```python
from build123d import *

# Parameters (mm, degrees)
BOSS_EXTRUDE1_DEPTH = 1.2
SKETCH2_W           = 8.848528138
SKETCH2_H           = 1.5
BOSS_EXTRUDE2_DEPTH = 1.2


with BuildPart() as part:
    # Sketch1 → Boss-Extrude1 (new body)
    with BuildSketch(Plane.XY):
        Polygon((4, 16.152543264), (-4, 16.152543264), (-20.152543264, 0), (0, -20.152543264), (20.152543264, 0), align=None)
        Polygon((-4.424264069, 16.152543264), (-4.624264069, 15.952543264), (-4.482842712, 15.952543264), (-20.435385976, 0), (0, -20.435385976), (20.435385976, 0), (4.482842712, 15.952543264), (4.624264069, 15.952543264), (4.424264069, 16.152543264), (4, 16.152543264), (20.152543264, 0), (0, -20.152543264), (-20.152543264, 0), (-4, 16.152543264), align=None)
        Polygon((-20.435385976, 0), (-4.482842712, 15.952543264), (-4.624264069, 15.952543264), (-20.576807333, 0), (0, -20.576807333), (20.576807333, 0), (4.624264069, 15.952543264), (4.482842712, 15.952543264), (20.435385976, 0), (0, -20.435385976), align=None)
    extrude(amount=BOSS_EXTRUDE1_DEPTH)

    # Sketch2 → Boss-Extrude2 (add)
    with BuildSketch(Plane.XY):
        with Locations((0, 16.902543264)):
            Rectangle(SKETCH2_W, SKETCH2_H)
    extrude(amount=BOSS_EXTRUDE2_DEPTH)


solid = part.part
```
Here's how the part is built. I have some questions about the finished solid (model axes, mm). A direction names the side the tool comes from. Coordinates: 2 decimals unless noted, no trailing zeros. Loops run counter-clockwise (first coordinate to the right, second up) from the corner with the lowest first, then second, coordinate; pieces in that order, holes last. Notation, with made-up numbers: (54.25, 4) - (85.25, 4) arc R20 ccw to (85.25, 10) - close; hole circle Ø7 at (27, 88.25). An arc over 180 degrees is marked (long way). Answer as CSV lines item,"result".
Q1. If I drill on L1, parallel to Y at x = -16.5, z = 0.95; L2, parallel to X at y = 14, z = 0.5; L3, parallel to Y at x = 10.5, z = 1.05, over which ranges is the centre line in solid material (lowest first)? Write a range as [from, to].
Response:
L1,"[-4.08, 4.08]"
L2,"[-6.58, 6.58]"
L3,"[-10.08, 10.08]"
Q2. If we section it at B-B, the plane y = 1: Write out the boundary of the cut face in (x, z), and give its area (3 significant figures).
Response:
outline,"(-19.58, 0) - (19.58, 0) - (19.58, 1.2) - (-19.58, 1.2) - close"
area,"47.0 mm2"
Q3. For faces 1 (the face through (-4.424, 17, 1)), 2 (the face through (0, -1, 0)), 3 (the face through (4.424, 17, 1)), which set-ups out of +Z, -Z, +X, -X, +Y, -Y let a thin tool reach every point of the face, with its end or its side?
Response:
face 1,"+Z, -Z, -X, +Y"
face 2,"-Z, +X, -X, +Y, -Y"
face 3,"+Z, -Z, +X, +Y"
Q4. If we section it at C-C, the plane x = 10: Write out the boundary of the cut face in (y, z).
Response:
outline,"(-10.58, 0) - (10.58, 0) - (10.58, 1.2) - (-10.58, 1.2) - close"
Q5. If we section it at A-A, the plane z = 0.7: Write out the boundary of the cut face in (x, y).
Response:
outline,"(-20.58, 0) - (0, -20.58) - (20.58, 0) - (4.42, 16.15) - (4.42, 17.65) - (-4.42, 17.65) - (-4.42, 16.15) - close"
Q6. For pin 1 (1.5 mm diameter, centred on x = 12.5, y = 9.5, fed in from +Z), with a flat end and sliding along its axis, tell me the tip position at first contact or that it passes through.
Response:
pin 1,"through"
